The listing builds one solid part. Answer for the finished solid, in the listing's coordinates (mm). Round coordinates to 2 decimals unless told otherwise and drop trailing zeros. Loops run counter-clockwise (first coordinate to the right, second up) from the corner with the lowest first, then second, coordinate; pieces in that order, holes last. Notation, with made-up numbers: M 51.5,-22 L 79.5,-22 A28 ccw 79.5,17 Z; hole C 37,82 d5. An arc over 180 degrees is marked long. Answer as a JSON object with one key per item and string values.
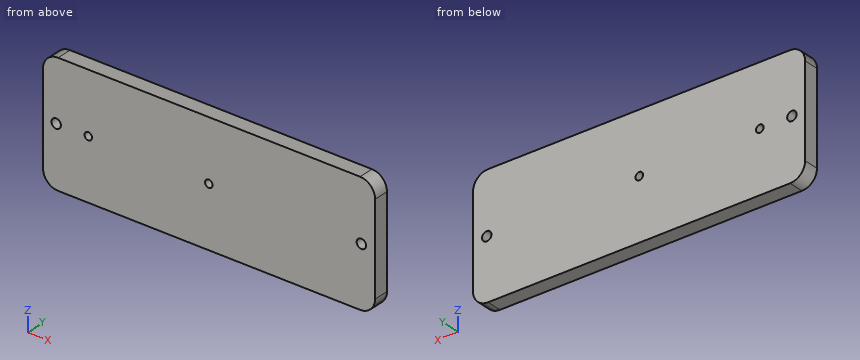
```python
from build123d import *

# Parameters (mm, degrees)
F1_DEPTH = 12.7
F3_D     = 7.9375
F5_D     = 6.35
F7_D     = 6.35


with BuildPart() as f1:
    # F0 (on Front) → F1 (new body)
    with BuildSketch(Plane.XZ):
        with BuildLine():
            Line((127.215293, 50.8), (-126.784707, 50.8))
            ThreePointArc((-126.784707, 50.8), (-135.764963, 47.080256), (-139.484707, 38.1))
            Line((-139.484707, 38.1), (-139.484707, -38.1))
            ThreePointArc((-139.484707, -38.1), (-135.764963, -47.080256), (-126.784707, -50.8))
            Line((-126.784707, -50.8), (127.215293, -50.8))
            ThreePointArc((127.215293, -50.8), (136.195549, -47.080256), (139.915293, -38.1))
            Line((139.915293, -38.1), (139.915293, 38.1))
            ThreePointArc((139.915293, 38.1), (136.195549, 47.080256), (127.215293, 50.8))
        make_face()
    extrude(amount=F1_DEPTH)

    # F3 (through all)
    with Locations(Plane.XZ.offset(12.7)):
        with Locations((-128.372207, 0), (128.372207, 0)):
            Hole(F3_D / 2)

    # F5 (through all)
    with Locations(Plane.XZ.offset(12.7)):
        with Locations((-101.384707, 0)):
            Hole(F5_D / 2)

    # F7 (through all)
    with Locations(Plane.XZ.offset(12.7)):
        with Locations((0, 0)):
            Hole(F7_D / 2)


solid = f1.part
```
Item 1: The part is cut by section B-B (x = 0). Give the vertices of the cut face in (y, z) (3 decimals).
Values follow:
{"outline": "M -12.7,-50.8 L 0,-50.8 L 0,-3.175 L -12.7,-3.175 Z; M -12.7,3.175 L 0,3.175 L 0,50.8 L -12.7,50.8 Z"}
Item 2: Straight lines are drawn through the part: line 1 (Z direction, x = 0, y = -5.5) (3 decimals); line 2 (X direction, y = -8, z = 41); line 3 (X direction, y = -4.75, z = -44). For each, find the intervals that lie inside material, in ascending order.
Values follow:
{"line 1": "-50.8 to -3.175, 3.175 to 50.8", "line 2": "-139.15 to 139.58", "line 3": "-138.03 to 138.46"}
Item 3: The part is cut by section A-A (z = 0). Give the vertices of the cut face in (x, y) (3 decimals), then the cut area to 3 significant figures.
Values follow:
{"outline": "M -139.485,-12.7 L -132.341,-12.7 L -132.341,0 L -139.485,0 Z; M -124.403,-12.7 L -104.56,-12.7 L -104.56,0 L -124.403,0 Z; M -98.21,-12.7 L -3.175,-12.7 L -3.175,0 L -98.21,0 Z; M 3.175,-12.7 L 124.403,-12.7 L 124.403,0 L 3.175,0 Z; M 132.341,-12.7 L 139.915,-12.7 L 139.915,0 L 132.341,0 Z", "area": "3,190 mm^2"}
Item 4: Flat-ended cylindrical pins translate along their axes: P1, Ø6.5, axis at x = 128.37, z = 0, coming from the -Y side; P2, Ø7.5, axis at x = 0, z = 0, coming from the -Y side. Find the tip coordinate at first contact, or state that the pin passes through.
Values follow:
{"P1": "through", "P2": "y = -12.7"}
